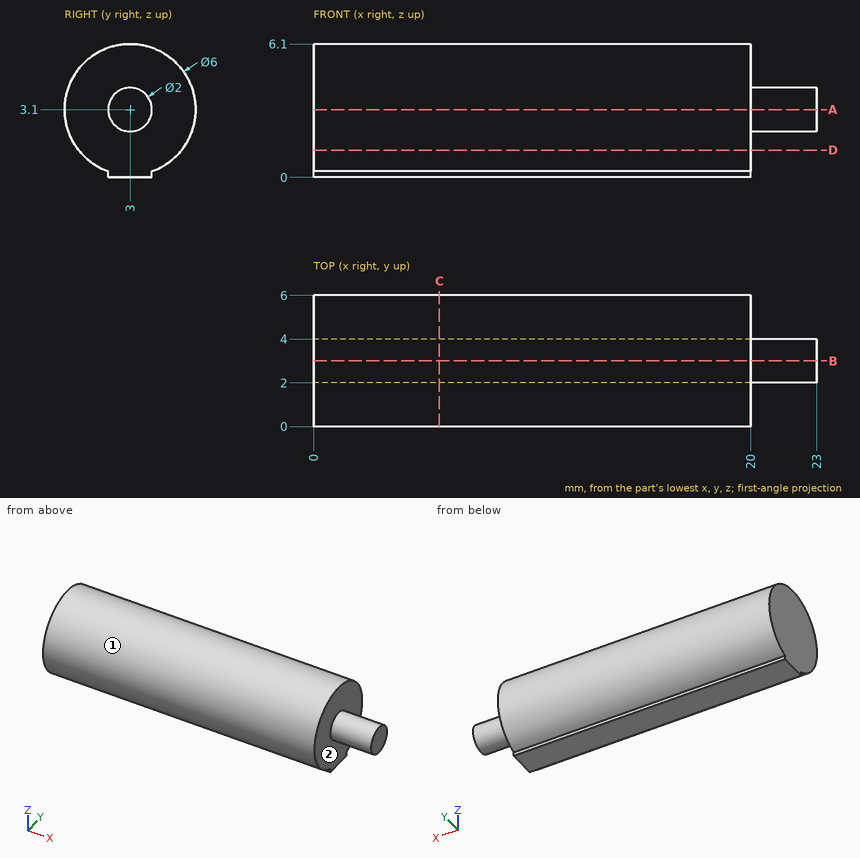
Source: three-view drawing plus pictorial views. Frame: mm from the lowest corner of the part. A direction names the side the tool comes from. Round coordinates to 2 decimals unless told otherwise and drop trailing zeros. Loops run counter-clockwise (first coordinate to the right, second up) from the corner with the lowest first, then second, coordinate; pieces in that order, holes last.
Q1. Access query for the marked faces 1 and 2. Directions: +Z, -Z, +X, -X, +Y, -Y. A direction counts if a zero-diameter tool reaches every point of the face in a straight line with its end or side. Return the directions, or none.
Q2. Material intervals for L1, parallel to X at y = 4.75, z = 3.75; L2, parallel to Y at x = 19, z = 3.25; L3, parallel to Z at x = 3.25, y = 2.5, sorted ascending.
Q3. Section B-B on y = 3. Return loops of the section in (x, z).
Q4. Section D-D on z = 1.25. Return loops of the section in (x, y), plus the area to 3 significant figures.
Q5. Pin query (flat end, axial travel): P1, Ø3, axis at x = 2.5, z = 4, coming from the -Y side; P2, Ø2, axis at x = 20, z = 1, coming from the +Y side. Return the tip coordinate at first contact, or that it passes through.
Q6. Section A-A on z = 3.1. Return loops of the section in (x, y), plus the area to 3 significant figures.
Q7. Section C-C on x = 5.75. Return loops of the section in (y, z), plus the area to 3 significant figures.
Evaluation:
1. face 1: +X, -X
1. face 2: +X
2. L1: x = 0 to 20
2. L2: y = 0 to 6
2. L3: z = 0 to 6.06
3. outline: (0, 0) - (20, 0) - (20, 2.1) - (23, 2.1) - (23, 4.1) - (20, 4.1) - (20, 6.1) - (0, 6.1) - close
4. outline: (0, 0.64) - (20, 0.64) - (20, 5.36) - (0, 5.36) - close
4. area: 94.5 mm2
5. P1: stops at y = 0
5. P2: stops at y = 5.79
6. outline: (0, 0) - (20, 0) - (20, 2) - (23, 2) - (23, 4) - (20, 4) - (20, 6) - (0, 6) - close
6. area: 126 mm2
7. outline: (2, 0) - (4, 0) - (4, 0.27) arc R3 ccw (long way) to (2, 0.27) - close
7. area: 28.6 mm2
